Can you work these out from the model? Positions are in its coordinate system, mm. A direction names the side the tool comes from. Coordinates: 2 decimals unless noted, no trailing zeros. Order: outer loops, then holes, each group sorted by start corner. A loop starts at its lowest first (then second) coordinate and runs counter-clockwise, first axis right, second up. Notation, with made-up numbers: (70.25, 79.25) -> (91.25, 79.25) arc R28 ccw to (91.25, 118.25) -> close; hole circle Ø4 at (49, 21). An arc over 180 degrees is marked (long way). Use a Markdown table: item, result. Add a question column.
1. For faces 1 (the flat face through (0, -0.75, 0)), 2 (the flat face through (-5.3, 3.1, 1.6)), which set-ups out of +Z, -Z, +X, -X, +Y, -Y let a thin tool reach every point of the face, with its end or its side?
2. Suppose I cut it at B-B, the plane z = 6. List the corners of the cut face in (x, y) for me.
3. Suppose I cut it at A-A, the plane y = 4.5. List the corners of the cut face in (x, z) for me (3 decimals), then the cut area to 3 significant figures.
4. If I drill on line 1 along X through (y, z) = (4, -4); line 2 along Z through (x, y) = (16, 4.5); line 3 along X through (y, z) = (4, 9), over which ranges is the centre line in solid material (lowest first)? Write a range as from..to.
5. For pin 1 Ø1.6 at (x, z) = (-5, 2) entering from +Y; pin 2 Ø2 at (x, z) = (-12, -7) entering from +Y, each with a flat end and sliding along its axis, tell me the tip position at first contact or that it passes through.
6. We'd pull the mould along Z, two halves only. Please class faces 3 (the flat face through (0, 3, 11.5)), 4 (the flat face through (-8, 6.1, -2)), 5 (the flat face through (5.3, 3.1, 1.6)): pulls with the +Z half, pulls with the -Z half, needs draft (parallel to the pull), parting line crosses it, or undercut.
7. Suppose I cut it at C-C, the plane x = 14. List the corners of the cut face in (y, z) for me, then the cut area to 3 significant figures.
8. Suppose I cut it at D-D, the plane z = -7. List the corners of the cut face in (x, y) for me, then the cut area to 3 significant figures.
```python
from build123d import *

# Parameters (mm, degrees)
SKETCH1_W           = 44
SKETCH1_H           = 23
BOSS_EXTRUDE1_DEPTH = 6
SKETCH2_W           = 44
SKETCH2_H           = 23
BOSS_EXTRUDE2_DEPTH = 0.75
CAVITY1_START       = 3
CAVITY1_OUTLINE_W   = 0.4
CAVITY1_OUTLINE_H   = 1.5
CAVITY1_OUTLINE_R   = 1.5
CAVITY1_DEPTH       = 3
CAVITY1_START_2     = 4
CAVITY1_2_OUTLINE_W = 0.4
CAVITY1_2_OUTLINE_H = 1.5
CAVITY1_2_DEPTH     = 2
CAVITY1_START_3     = 3.1
CAVITY1_3_OUTLINE_W = 0.4
CAVITY1_3_OUTLINE_H = 1.5
CAVITY1_3_DEPTH     = 0.9
CAVITY1_START_4     = 3.5
CAVITY1_4_DEPTH     = 0.5
SKETCH5_R           = 1.5
SKETCH5_R_2         = 0.35
BOSS_EXTRUDE3_DEPTH = 0.1


# Read off the part's stored shape, not the designer's step: Cavity1
with BuildPart() as part:
    # Sketch1 → Boss-Extrude1 (new body)
    with BuildSketch(Plane(origin=(0, 0, 0), x_dir=(1, 0, 0), z_dir=(0, 1, 0))):
        Rectangle(SKETCH1_W, SKETCH1_H)
    extrude(amount=BOSS_EXTRUDE1_DEPTH)

    # Sketch2 → Boss-Extrude2 (add)
    with BuildSketch(Plane.XZ):
        Rectangle(SKETCH2_W, SKETCH2_H)
    extrude(amount=BOSS_EXTRUDE2_DEPTH)

    # Cavity1 outline → Cavity1 (cut)
    with BuildSketch(Plane(origin=(0, 0, 0), x_dir=(1, 0, 0), z_dir=(0, 1, 0)).offset(CAVITY1_START)):
        Polygon((20, -9.5), (20, 5.5), (11.824003475, 5.5), (5.87, 9.5), (-5.87, 9.5), (-11.824003475, 5.5), (-20, 5.5), (-20, -9.5), align=None)
        with Locations((-6.57, -1.65)):
            Rectangle(CAVITY1_OUTLINE_W, CAVITY1_OUTLINE_H, mode=Mode.SUBTRACT)
        Polygon((-5.87, -2.4), (-5.87, -0.9), (-4.37, -1.65), align=None, mode=Mode.SUBTRACT)
        Polygon((4.37, -1.65), (5.87, -0.9), (5.87, -2.4), align=None, mode=Mode.SUBTRACT)
        with Locations((6.57, -1.65)):
            Rectangle(CAVITY1_OUTLINE_W, CAVITY1_OUTLINE_H, mode=Mode.SUBTRACT)
        with Locations((-8, 1.565)):
            Circle(CAVITY1_OUTLINE_R, mode=Mode.SUBTRACT)
        Polygon((-4.37, 5.5), (-5.87, 4.75), (-5.87, 6.25), align=None, mode=Mode.SUBTRACT)
        with Locations((8, 1.565)):
            Circle(CAVITY1_OUTLINE_R, mode=Mode.SUBTRACT)
        with BuildLine():
            ThreePointArc((-3.0745499, 2.214515103), (-3.36304333, 1.678756458), (-3.67597558, 2.200617734))
            Line((-3.67597558, 2.200617734), (-3.084051452, 3.25))
            Line((-3.084051452, 3.25), (3.084051452, 3.25))
            Line((3.084051452, 3.25), (3.67597558, 2.200617734))
            ThreePointArc((3.67597558, 2.200617734), (3.36304333, 1.678756458), (3.0745499, 2.214515103))
            Line((3.0745499, 2.214515103), (2.698000841, 2.95))
            Line((2.698000841, 2.95), (-2.698000841, 2.95))
            Line((-2.698000841, 2.95), (-3.0745499, 2.214515103))
        make_face(mode=Mode.SUBTRACT)
        with BuildLine():
            ThreePointArc((3.039420657, 4), (3.614959604, 4.314575131), (3.385830819, 3.7))
            Line((3.385830819, 3.7), (-3.385830819, 3.7))
            ThreePointArc((-3.385830819, 3.7), (-3.614959604, 4.314575131), (-3.039420657, 4))
            Line((-3.039420657, 4), (3.039420657, 4))
        make_face(mode=Mode.SUBTRACT)
        Polygon((4.37, 5.5), (5.87, 6.25), (5.87, 4.75), align=None, mode=Mode.SUBTRACT)
    extrude(amount=CAVITY1_DEPTH, mode=Mode.SUBTRACT)

    # Cavity1 2 outline → Cavity1 2 (cut)
    with BuildSketch(Plane(origin=(0, 0, 0), x_dir=(1, 0, 0), z_dir=(0, 1, 0)).offset(CAVITY1_START_2)):
        Polygon((20, 5.5), (20, 9.5), (5.87, 9.5), (11.824003475, 5.5), align=None)
        Polygon((-11.824003475, 5.5), (-5.87, 9.5), (-20, 9.5), (-20, 5.5), align=None)
        with BuildLine():
            ThreePointArc((3.385830819, 3.7), (3.156702034, 3.785424869), (3.039420657, 4))
            Line((3.039420657, 4), (-3.039420657, 4))
            ThreePointArc((-3.039420657, 4), (-3.156702034, 3.785424869), (-3.385830819, 3.7))
            Line((-3.385830819, 3.7), (3.385830819, 3.7))
        make_face()
        with BuildLine():
            ThreePointArc((-3.67597558, 2.200617734), (-3.379214176, 2.37856965), (-3.0745499, 2.214515103))
            Line((-3.0745499, 2.214515103), (-2.698000841, 2.95))
            Line((-2.698000841, 2.95), (2.698000841, 2.95))
            Line((2.698000841, 2.95), (3.0745499, 2.214515103))
            ThreePointArc((3.0745499, 2.214515103), (3.379214176, 2.37856965), (3.67597558, 2.200617734))
            Line((3.67597558, 2.200617734), (3.084051452, 3.25))
            Line((3.084051452, 3.25), (-3.084051452, 3.25))
            Line((-3.084051452, 3.25), (-3.67597558, 2.200617734))
        make_face()
        Polygon((5.87, 4.75), (5.87, 6.25), (4.37, 5.5), align=None)
        Polygon((5.87, -2.4), (5.87, -0.9), (4.37, -1.65), align=None)
        Polygon((-4.37, -1.65), (-5.87, -0.9), (-5.87, -2.4), align=None)
        Polygon((-5.87, 6.25), (-5.87, 4.75), (-4.37, 5.5), align=None)
        with Locations((-6.57, -1.65)):
            Rectangle(CAVITY1_2_OUTLINE_W, CAVITY1_2_OUTLINE_H)
        with Locations((6.57, -1.65)):
            Rectangle(CAVITY1_2_OUTLINE_W, CAVITY1_2_OUTLINE_H)
    extrude(amount=CAVITY1_2_DEPTH, mode=Mode.SUBTRACT)

    # Cavity1 3 outline → Cavity1 3 (cut)
    with BuildSketch(Plane(origin=(0, 0, 0), x_dir=(1, 0, 0), z_dir=(0, 1, 0)).offset(CAVITY1_START_3)):
        Polygon((5.87, 4.75), (5.87, 6.25), (4.37, 5.5), align=None)
        Polygon((5.87, -2.4), (5.87, -0.9), (4.37, -1.65), align=None)
        Polygon((-4.37, -1.65), (-5.87, -0.9), (-5.87, -2.4), align=None)
        Polygon((-5.87, 6.25), (-5.87, 4.75), (-4.37, 5.5), align=None)
        with Locations((-6.57, -1.65)):
            Rectangle(CAVITY1_3_OUTLINE_W, CAVITY1_3_OUTLINE_H)
        with Locations((6.57, -1.65)):
            Rectangle(CAVITY1_3_OUTLINE_W, CAVITY1_3_OUTLINE_H)
    extrude(amount=CAVITY1_3_DEPTH, mode=Mode.SUBTRACT)

    # Cavity1 4 outline → Cavity1 4 (cut)
    with BuildSketch(Plane(origin=(0, 0, 0), x_dir=(1, 0, 0), z_dir=(0, 1, 0)).offset(CAVITY1_START_4)):
        with BuildLine():
            ThreePointArc((3.385830819, 3.7), (3.156702034, 3.785424869), (3.039420657, 4))
            Line((3.039420657, 4), (-3.039420657, 4))
            ThreePointArc((-3.039420657, 4), (-3.156702034, 3.785424869), (-3.385830819, 3.7))
            Line((-3.385830819, 3.7), (3.385830819, 3.7))
        make_face()
        with BuildLine():
            ThreePointArc((-3.67597558, 2.200617734), (-3.379214176, 2.37856965), (-3.0745499, 2.214515103))
            Line((-3.0745499, 2.214515103), (-2.698000841, 2.95))
            Line((-2.698000841, 2.95), (2.698000841, 2.95))
            Line((2.698000841, 2.95), (3.0745499, 2.214515103))
            ThreePointArc((3.0745499, 2.214515103), (3.379214176, 2.37856965), (3.67597558, 2.200617734))
            Line((3.67597558, 2.200617734), (3.084051452, 3.25))
            Line((3.084051452, 3.25), (-3.084051452, 3.25))
            Line((-3.084051452, 3.25), (-3.67597558, 2.200617734))
        make_face()
    extrude(amount=CAVITY1_4_DEPTH, mode=Mode.SUBTRACT)

    # Sketch5 → Boss-Extrude3 (add)
    with BuildSketch(Plane(origin=(0, 6, 0), x_dir=(1, 0, 0), z_dir=(0, 1, 0))):
        with Locations(Location((-8, 1.565, 0), (0, 0, 270))):
            Circle(SKETCH5_R)
        with Locations(Location((8, 1.565, 0), (0, 0, 270))):
            Circle(SKETCH5_R)
        with Locations(Location((-3.385830819, 4.05, 0), (0, 0, 270))):
            Circle(SKETCH5_R_2)
        with Locations(Location((-3.371128753, 2.028663054, 0), (0, 0, 32.073441705))):
            Circle(SKETCH5_R_2)
        with Locations(Location((3.385830819, 4.05, 0), (0, 0, 270))):
            Circle(SKETCH5_R_2)
        with Locations(Location((3.371128753, 2.028663054, 0), (0, 0, 147.926558295))):
            Circle(SKETCH5_R_2)
    extrude(amount=BOSS_EXTRUDE3_DEPTH)


solid = part.part
```
Worked out:
| question | item | result |
|---|---|---|
| 1 | face 1 | +Z, -Z, +X, -X, -Y |
| 1 | face 2 | +Y |
| 2 | outline | (-22, -0.75) -> (22, -0.75) -> (22, 6) -> (20, 6) -> (20, 3) -> (-20, 3) -> (-20, 6) -> (-22, 6) -> close |
| 3 | outline | (-22, -11.5) -> (22, -11.5) -> (22, 11.5) -> (-22, 11.5) -> close; circle Ø3 at (-8, -1.565); circle Ø0.7 at (-3.386, -4.05); circle Ø0.7 at (-3.371, -2.029); circle Ø0.7 at (3.371, -2.029); circle Ø0.7 at (3.386, -4.05); circle Ø3 at (8, -1.565); hole (-20, -9.5) -> (20, -9.5) -> (20, 9.5) -> (-20, 9.5) -> close |
| 3 | area | 268 mm² |
| 4 | line 1 | x = -22..-20, -3.73..-3.04, 3.04..3.73, 20..22 |
| 4 | line 2 | z = -11.5..-9.5, 9.5..11.5 |
| 4 | line 3 | x = -22..-20, 20..22 |
| 5 | pin 1 | stops at y = 3.1 |
| 5 | pin 2 | stops at y = 4 |
| 6 | face 3 | pulls with the +Z half |
| 6 | face 4 | needs draft |
| 6 | face 5 | undercut |
| 7 | outline | (-0.75, -11.5) -> (6, -11.5) -> (6, -9.5) -> (4, -9.5) -> (4, -5.5) -> (3, -5.5) -> (3, 9.5) -> (6, 9.5) -> (6, 11.5) -> (-0.75, 11.5) -> close |
| 7 | area | 102 mm² |
| 8 | outline | (-22, -0.75) -> (22, -0.75) -> (22, 6) -> (20, 6) -> (20, 4) -> (9.59, 4) -> (9.59, 3) -> (-9.59, 3) -> (-9.59, 4) -> (-20, 4) -> (-20, 6) -> (-22, 6) -> close |
| 8 | area | 198 mm² |
